Input: part model. Units: mm. Frame: model coordinates. Face numbers are marked on the shaded views. A direction names the side the tool comes from. Coordinates: 2 decimals unless noted, no trailing zeros. Order: outer loops, then holes, each group sorted by start corner. A loop starts at its lowest first (then second) coordinate and runs counter-clockwise, first axis right, second up. Notation, with made-up numbers: (28.25, 34) - (44.25, 34) arc R15 ccw to (44.25, 45) - close; hole circle Ø3 at (-6.75, 55). An arc over 180 degrees is marked (long way). Use a Markdown table: item, result. Add a question column.
from build123d import *

# Parameters (mm, degrees)
F0_W      = 101.6
F0_H      = 10.6841248744
F1_DEPTH  = 76.2
F2_W      = 101.6
F2_H      = 10.6841248744
F2_H_2    = 76.766988388
F3_DEPTH  = 8.6953
F5_DEPTH  = 76.2
F6_W      = 94.0149463713
F6_H      = 46.6581489891
F7_DEPTH  = 10.16
F9_DEPTH  = 67.5047
F11_DEPTH = 6.35
F12_W     = 83.7408676744
F12_H     = 77.5378420949
F13_DEPTH = 76.201
F15_DEPTH = 12.7


with BuildPart() as f1:
    # F0 (on Front) → F1 (new body)
    with BuildSketch(Plane.XZ):
        with Locations((2.113474533, -32.5691830367)):
            Rectangle(F0_W, F0_H)
    extrude(amount=F1_DEPTH)

    # F2 (on Front) → F3 (join)
    with BuildSketch(Plane.XZ):
        with Locations((2.113474533, -32.5691830367)):
            Rectangle(F2_W, F2_H)
        with Locations((2.113474533, 11.1563735945)):
            Rectangle(F2_W, F2_H_2)
    extrude(amount=F3_DEPTH)

    # F4 (on Front) → F5 (join)
    with BuildSketch(Plane.XZ):
        Polygon((2.113474533, 105.0908565521), (-48.686525467, 49.5398677886), (52.913474533, 49.5398677886), align=None)
    extrude(amount=F5_DEPTH)

    # F6 (on face) → F7 (cut)
    with BuildSketch(Plane.XY.offset(-27.2271205995)):
        with Locations((2.4187173694, -42.054575868)):
            Rectangle(F6_W, F6_H)
    extrude(amount=-F7_DEPTH, mode=Mode.SUBTRACT)

    # F8 (on face) → F9 (cut, through all)
    with BuildSketch(Plane.XZ.offset(76.2)):
        Polygon((0, 91.7181875073), (-38.5710261762, 49.5398677886), (46.1229796213, 49.5398677886), align=None)
    extrude(amount=-F9_DEPTH, mode=Mode.SUBTRACT)

    # F10 (on face) → F11 (join)
    with BuildSketch(Plane.XZ.offset(76.2)):
        Polygon((0, 91.7181875073), (-38.5710261762, 49.5398677886), (46.1229796213, 49.5398677886), align=None)
    extrude(amount=-F11_DEPTH)

    # F12 (on Front) → F13 (cut, through all)
    with BuildSketch(Plane.XZ):
        with Locations((1.9384473562, 9.5993131399)):
            Rectangle(F12_W, F12_H)
    extrude(amount=F13_DEPTH, mode=Mode.SUBTRACT)

    # F14 (on face) → F15 (cut)
    with BuildSketch(Plane(origin=(0, 0, 0), x_dir=(-1, 0, 0), z_dir=(0, 1, 0))):
        Polygon((0, 91.7181875073), (-43.8088811934, 48.3682341874), (39.931986481, 48.3682341874), align=None)
    extrude(amount=-F15_DEPTH, mode=Mode.SUBTRACT)


solid = f1.part
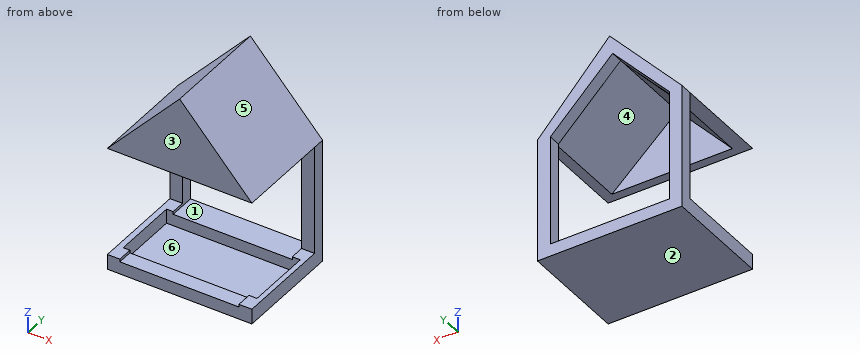
1) Cut plane B-B (z = 19.5). Return the cut outline in (x, y), and give its area (3 significant figures).
2) Cut plane C-C (x = 15). Return the cut outline in (y, z).
3) Contact query for flat-ended pins moving along their axis: P1, Ø6, axis at x = -25.5, z = 61, coming from the +Y side; P2, Ø3, axis at y = -48.5, z = 59, coming from the -X side; P3, Ø4.5, axis at x = 48, y = -55.5, coming from the +Z side; P4, Ø4.5, axis at x = -46, y = -54.5, coming from the +Z side. Output: stop coordinate, or through.
4) Cut plane A-A (y = -39.5). Return the cut outline in (x, z).
5) Material intervals for L1, parallel to Y at x = 3, z = 56.5; L2, parallel to Z at x = 3, y = -14; L3, parallel to Z at x = -36.5, y = -67, sorted ascending.
6) Pull-direction query (Y, two-part tool) for the marked faces 3, 4, 5 and 6; classes: pulls with the +Y half, pulls with the -Y half, needs draft (parallel to the pull), parting line crosses it, or undercut.
7) Reachability of the marked faces 1 and 2 from +Z, -Z, +X, -X, +Y, -Y: full face, straight path, thin tool, end or side. Return the list, or none.
8) Cut plane D-D (x = 37.5). Return the cut outline in (y, z).
Computed:
| question | item | result |
|---|---|---|
| 1 | outline | (-48.69, -8.7) - (-39.93, -8.7) - (-39.93, 0) - (-48.69, 0) - close; (43.81, -8.7) - (52.91, -8.7) - (52.91, 0) - (43.81, 0) - close |
| 1 | area | 155 mm2 |
| 2 | outline | (-76.2, -37.91) - (0, -37.91) - (0, -29.17) - (-18.73, -29.17) - (-18.73, -37.39) - (-65.38, -37.39) - (-65.38, -29.17) - (-76.2, -29.17) - close; (-76.2, 49.54) - (-69.85, 49.54) - (-69.85, 78) - (-8.7, 78) - (-8.7, 76.88) - (0, 76.88) - (0, 91) - (-76.2, 91) - close |
| 3 | P1 | stops at y = 0 |
| 3 | P2 | stops at x = -41.41 |
| 3 | P3 | stops at z = 57.37 |
| 3 | P4 | stops at z = 54.94 |
| 4 | outline | (-48.69, -37.91) - (52.91, -37.91) - (52.91, -27.23) - (49.43, -27.23) - (49.43, -37.39) - (-44.59, -37.39) - (-44.59, -27.23) - (-48.69, -27.23) - close; (-48.69, 49.54) - (-38.57, 49.54) - (0, 91.72) - (46.12, 49.54) - (52.91, 49.54) - (2.11, 105.09) - close |
| 5 | L1 | y = -76.2 to -69.85 |
| 5 | L2 | z = -37.91 to -29.17, 88.97 to 104.12 |
| 5 | L3 | z = -37.91 to -29.17, 51.8 to 62.87 |
| 6 | face 3 | pulls with the -Y half |
| 6 | face 4 | undercut |
| 6 | face 5 | needs draft |
| 6 | face 6 | undercut |
| 7 | face 1 | +Y, -Y |
| 7 | face 2 | -Z, +X, -X, +Y, -Y |
| 8 | outline | (-76.2, -37.91) - (0, -37.91) - (0, -29.17) - (-18.73, -29.17) - (-18.73, -37.39) - (-65.38, -37.39) - (-65.38, -29.17) - (-76.2, -29.17) - close; (-76.2, 49.54) - (-69.85, 49.54) - (-69.85, 57.43) - (-8.7, 57.43) - (-8.7, 54.61) - (0, 54.61) - (0, 66.39) - (-76.2, 66.39) - close |
